Job drawing, mm, ordinate dimensions from the low corner. One solid piece. A direction names the side the tool comes from. Give positions to 0.01 mm unless a question says otherwise; leave off trailing zeros. Order: outer loops, then holes, each group sorted by start corner. A loop starts at its lowest first (then second) coordinate and runs counter-clockwise, first axis right, second up.
Item 1: Wall check: L1, parallel to X at y = 5.25, z = 19.5; L2, parallel to Y at x = 27, z = 13.75; L3, parallel to X at y = 19.25, z = 18. Give the ranges that are in metal, low to high.
Item 2: Band-saw the part on A-A on z = 14.05. Give the cut face in (x, y).
Item 3: Band-saw the part on D-D on y = 22. Give the cut face in (x, z), plus the area to 3 significant figures.
Item 4: Flat gauge pins, fed straight in: P1, Ø2, axis at x = 50.5, z = 10, coming from the +Y side; P2, Ø6, axis at x = 40, y = 4.5, coming from the -Z side; P3, Ø1.5, axis at y = 13, z = 19.5, coming from the +X side; P4, Ø1.5, axis at x = 17, z = 25, coming from the -Y side. Where does each tip first touch, or does it go through?
Item 5: Band-saw the part on C-C on x = 7. Give the cut face in (y, z), plus the area to 3 significant figures.
Item 6: Which spindle directions (+Z, -Z, +X, -X, +Y, -Y) get a long thin tool onto all of the face, cutting with end or side? Do the marked faces 1, 2 and 3. Say none if no direction does.
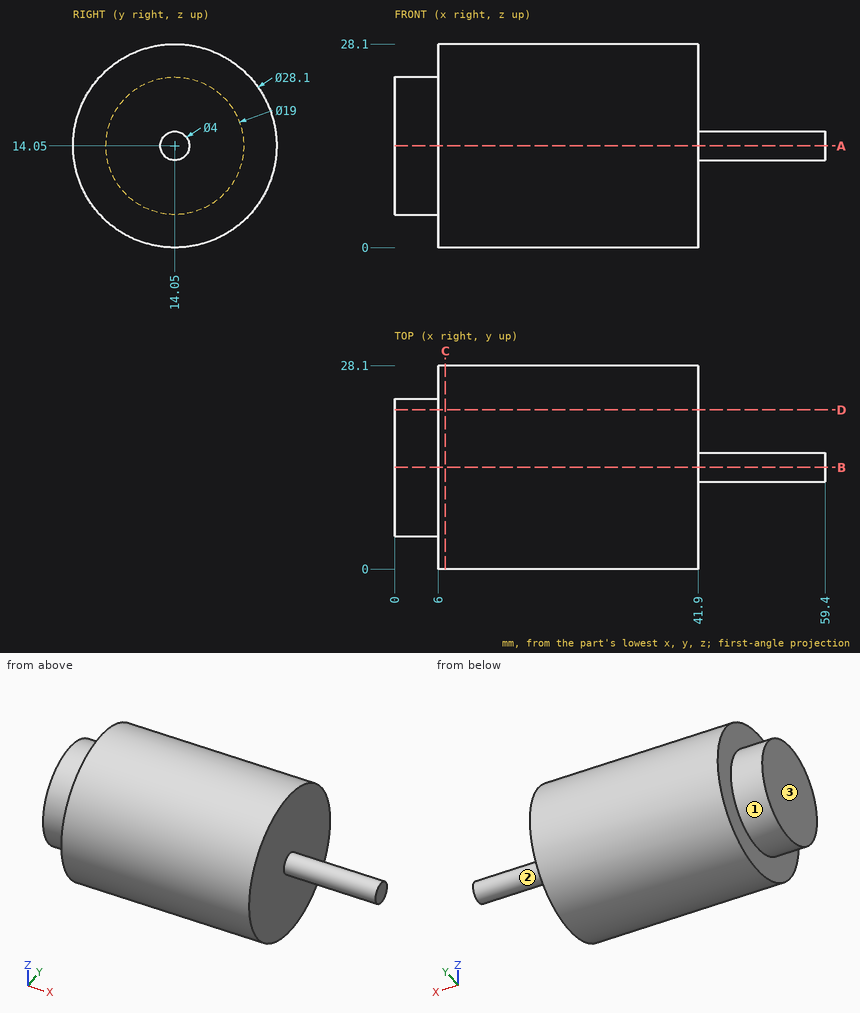
The answers:
1. L1: x = 6 to 41.9
1. L2: y = 0 to 28.1
1. L3: x = 0 to 41.9
2. outline: (0, 4.55) - (6, 4.55) - (6, 0) - (41.9, 0) - (41.9, 12.05) - (59.4, 12.05) - (59.4, 16.05) - (41.9, 16.05) - (41.9, 28.1) - (6, 28.1) - (6, 23.55) - (0, 23.55) - close
3. outline: (0, 8.85) - (6, 8.85) - (6, 2.47) - (41.9, 2.47) - (41.9, 25.63) - (6, 25.63) - (6, 19.25) - (0, 19.25) - close
3. area: 894 mm2
4. P1: passes through
4. P2: stops at z = 1.62
4. P3: stops at x = 41.9
4. P4: stops at y = 4.39
5. outline: circle Ø28.1 at (14.05, 14.05)
5. area: 620 mm2
6. face 1: -X
6. face 2: +X
6. face 3: +Z, -Z, -X, +Y, -Y
